Work out the finished part from the listing and answer in its coordinate system (mm). A direction names the side the tool comes from. Coordinates: 2 decimals unless noted, no trailing zeros. Order: outer loops, then holes, each group sorted by start corner. A loop starts at its lowest first (then second) coordinate and runs counter-clockwise, first axis right, second up. Notation, with made-up numbers: M -23.75,82 L 9.25,82 A19 cw 9.25,97 Z; hole C -19,31 d8. An arc over 180 degrees is marked long. Use a Markdown table: item, result. Add a question column.
from build123d import *

# Parameters (mm, degrees)
SKETCH1_W                                  = 200
SKETCH1_H                                  = 400
BOSS_EXTRUDE1_DEPTH                        = 60
SKETCH2_R                                  = 15
CUT_EXTRUDE1_DEPTH                         = 452.220566907
SKETCH3_W                                  = 30
SKETCH3_H                                  = 90
CUT_EXTRUDE2_DEPTH                         = 452.220566907
MIRROR1_AT_THE_SECOND_PLANE_COPY_1_SKETC_W = 30
MIRROR1_AT_THE_SECOND_PLANE_COPY_1_SKETC_H = 90
MIRROR1_AT_THE_SECOND_PLANE_COPY_1_DEPTH   = 452.220566907
FILLET1_R                                  = 10
FILLET2_R                                  = 10


with BuildPart() as part:
    # Sketch1 → Boss-Extrude1 (new body)
    with BuildSketch(Plane.XY):
        with Locations((100, 200)):
            Rectangle(SKETCH1_W, SKETCH1_H)
    extrude(amount=BOSS_EXTRUDE1_DEPTH)

    # Sketch2 → Cut-Extrude1 (cut, through all)
    with BuildSketch(Plane(origin=(200, 0, 0), x_dir=(0, 0, -1), z_dir=(1, 0, 0))):
        with Locations(Location((-30, 40, 0), (0, 0, 90))):
            Circle(SKETCH2_R)
        with Locations(Location((-30, 360, 0), (0, 0, 90))):
            Circle(SKETCH2_R)
    extrude(amount=-CUT_EXTRUDE1_DEPTH, mode=Mode.SUBTRACT)

    # Sketch3 → Cut-Extrude2 (cut, through all)
    with BuildSketch(Plane(origin=(0, 0, 0), x_dir=(-1, 0, 0), z_dir=(0, 0, -1))):
        with Locations((-15, 45)):
            Rectangle(SKETCH3_W, SKETCH3_H)
    cut_extrude2 = extrude(amount=-CUT_EXTRUDE2_DEPTH, mode=Mode.SUBTRACT)

    # Mirror1: Cut-Extrude2 across plane
    add(cut_extrude2.mirror(Plane(origin=(100, 0, 0), x_dir=(0, 0, 1), z_dir=(1, 0, 0))), mode=Mode.SUBTRACT)

    # Mirror1 at the second plane: Cut-Extrude2 across plane
    add(cut_extrude2.mirror(Plane.ZX.offset(200)), mode=Mode.SUBTRACT)

    # Mirror1 at the second plane copy 1 sketc → Mirror1 at the second plane copy 1 (cut, through all)
    with BuildSketch(Plane(origin=(200, 400, 0), x_dir=(1, 0, 0), z_dir=(0, 0, -1))):
        with Locations((-15, 45)):
            Rectangle(MIRROR1_AT_THE_SECOND_PLANE_COPY_1_SKETC_W, MIRROR1_AT_THE_SECOND_PLANE_COPY_1_SKETC_H)
    extrude(amount=-MIRROR1_AT_THE_SECOND_PLANE_COPY_1_DEPTH, mode=Mode.SUBTRACT)

    # Fillet1
    fillet1_edges = [part.edges().sort_by_distance(p)[0] for p in [
        (100, 0, 0),
        (0, 90, 30),
        (30, 45, 60),
        (30, 0, 30),
        (15, 90, 60),
        (15, 90, 0),
        (30, 45, 0),
        (0, 200, 0),
        (0, 200, 60),
        (30, 355, 0),
        (15, 310, 0),
        (0, 310, 30),
        (30, 400, 30),
        (15, 310, 60),
        (30, 355, 60),
        (100, 400, 0),
    ]]
    fillet(fillet1_edges, radius=FILLET1_R)

    # Fillet2
    # the kernel refuses this fillet: 10 mm, written as the material it takes off along each edge
    with BuildSketch(Plane(origin=(40, 10, 50), x_dir=(0, -1, 0), z_dir=(0, 0, 1))) as fillet2_piece_1_section:
        Polygon((0, 0), (FILLET2_R, 0), (FILLET2_R, -FILLET2_R), (0, -FILLET2_R), align=None)
    fillet2_piece_1 = extrude(amount=FILLET2_R, mode=Mode.PRIVATE)
    fillet2_piece_1 = fillet2_piece_1 - Plane(origin=(40, 10, 50), x_dir=(0.7071067811865476, 0.7071067811865475, 0), z_dir=(0, 0, 1)) * Sphere(FILLET2_R, mode=Mode.PRIVATE)
    add(fillet2_piece_1, mode=Mode.SUBTRACT)
    with BuildSketch(Plane(origin=(190, 300, 50), x_dir=(1, 0, 0), z_dir=(0, 0, 1))) as fillet2_piece_2_section:
        Polygon((0, 0), (FILLET2_R, 0), (FILLET2_R, FILLET2_R), (0, FILLET2_R), align=None)
    fillet2_piece_2 = extrude(amount=FILLET2_R, mode=Mode.PRIVATE)
    fillet2_piece_2 = fillet2_piece_2 - Plane(origin=(190, 300, 50), x_dir=(-0.7071067811865471, -0.707106781186548, 0), z_dir=(0, 0, 1)) * Sphere(FILLET2_R, mode=Mode.PRIVATE)
    add(fillet2_piece_2, mode=Mode.SUBTRACT)
    with BuildSketch(Plane(origin=(190, 100, 50), x_dir=(0, -1, 0), z_dir=(0, 0, 1))) as fillet2_piece_3_section:
        Polygon((0, 0), (FILLET2_R, 0), (FILLET2_R, FILLET2_R), (0, FILLET2_R), align=None)
    fillet2_piece_3 = extrude(amount=FILLET2_R, mode=Mode.PRIVATE)
    fillet2_piece_3 = fillet2_piece_3 - Plane(origin=(190, 100, 50), x_dir=(-0.7071067811865472, 0.7071067811865478, 0), z_dir=(0, 0, 1)) * Sphere(FILLET2_R, mode=Mode.PRIVATE)
    add(fillet2_piece_3, mode=Mode.SUBTRACT)
    with BuildSketch(Plane(origin=(160, 10, 50), x_dir=(0, -1, 0), z_dir=(1, 0, 0))) as fillet2_piece_4_section:
        Polygon((0, 0), (FILLET2_R, 0), (FILLET2_R, -FILLET2_R), (0, -FILLET2_R), align=None)
    fillet2_piece_4 = extrude(amount=FILLET2_R, mode=Mode.PRIVATE)
    fillet2_piece_4 = fillet2_piece_4 - Plane(origin=(160, 10, 50), x_dir=(0, 0.7071067811865475, -0.7071067811865475), z_dir=(1, 0, 0)) * Sphere(FILLET2_R, mode=Mode.PRIVATE)
    add(fillet2_piece_4, mode=Mode.SUBTRACT)
    with BuildSketch(Plane(origin=(170, 10, 10), x_dir=(0, 0, -1), z_dir=(0, 1, 0))) as fillet2_piece_5:
        with BuildLine():
            CenterArc((10 - FILLET2_R, FILLET2_R), FILLET2_R, 270, 90)
            Line((10, FILLET2_R), (10, 0))
            Line((10, 0), (10 - FILLET2_R, 0))
        make_face()
    revolve(axis=Axis((170, 10, 10), (-1, 0, 0)), revolution_arc=90, mode=Mode.SUBTRACT)
    with BuildSketch(Plane(origin=(170, 390, 10), x_dir=(0, 0, -1), z_dir=(0, -1, 0))) as fillet2_piece_6:
        with BuildLine():
            CenterArc((10 - FILLET2_R, -FILLET2_R), FILLET2_R, 0, 90)
            Line((10, -FILLET2_R), (10, 0))
            Line((10, 0), (10 - FILLET2_R, 0))
        make_face()
    revolve(axis=Axis((170, 390, 10), (1, 0, 0)), revolution_arc=90, mode=Mode.SUBTRACT)
    with BuildSketch(Plane(origin=(200, 335, 0), x_dir=(-1, 0, 0), z_dir=(0, -1, 0))) as fillet2_piece_7:
        with BuildLine():
            CenterArc((FILLET2_R, -FILLET2_R), FILLET2_R, 90, 90)
            Line((0, -FILLET2_R), (0, 0))
            Line((0, 0), (FILLET2_R, 0))
        make_face()
    extrude(amount=270, mode=Mode.SUBTRACT)
    with BuildSketch(Plane(origin=(200, 300, 60), x_dir=(-1, 0, 0), z_dir=(0, -1, 0))) as fillet2_piece_8:
        with BuildLine():
            CenterArc((FILLET2_R, FILLET2_R), FILLET2_R, 180, 90)
            Line((0, FILLET2_R), (0, 0))
            Line((0, 0), (FILLET2_R, 0))
        make_face()
    extrude(amount=200, mode=Mode.SUBTRACT)
    with BuildSketch(Plane(origin=(170, 90, 0), x_dir=(-1, 0, 0), z_dir=(0, -1, 0))) as fillet2_piece_9:
        with BuildLine():
            CenterArc((FILLET2_R, -FILLET2_R), FILLET2_R, 90, 90)
            Line((0, -FILLET2_R), (0, 0))
            Line((0, 0), (FILLET2_R, 0))
        make_face()
    extrude(amount=80, mode=Mode.SUBTRACT)
    with BuildSketch(Plane(origin=(200, 90, -25), x_dir=(-1, 0, 0), z_dir=(0, 0, 1)), Plane(origin=(200, 310, -25), x_dir=(0, -1, 0), z_dir=(0, 0, 1)), Plane(origin=(170, 400, 10), x_dir=(0, -1, 0), z_dir=(0, 0, 1))) as fillet2_piece_10:
        with BuildLine():
            CenterArc((FILLET2_R, -FILLET2_R), FILLET2_R, 90, 90)
            Line((0, -FILLET2_R), (0, 0))
            Line((0, 0), (FILLET2_R, 0))
        make_face()
    extrude(amount=75, mode=Mode.SUBTRACT)
    with BuildSketch(Plane(origin=(170, 0, 10), x_dir=(0, 1, 0), z_dir=(0, 0, 1))) as fillet2_piece_11:
        with BuildLine():
            CenterArc((FILLET2_R, FILLET2_R), FILLET2_R, 180, 90)
            Line((0, FILLET2_R), (0, 0))
            Line((0, 0), (FILLET2_R, 0))
        make_face()
    extrude(amount=40, mode=Mode.SUBTRACT)
    with BuildSketch(Plane(origin=(190, 90, 60), x_dir=(0, 1, 0), z_dir=(-1, 0, 0))) as fillet2_piece_12:
        with BuildLine():
            CenterArc((FILLET2_R, FILLET2_R), FILLET2_R, 180, 90)
            Line((0, FILLET2_R), (0, 0))
            Line((0, 0), (FILLET2_R, 0))
        make_face()
    extrude(amount=20, mode=Mode.SUBTRACT)
    with BuildSketch(Plane(origin=(170, 90, 60), x_dir=(-1, 0, 0), z_dir=(0, -1, 0)), Plane(origin=(170, 310, 0), x_dir=(-1, 0, 0), z_dir=(0, 1, 0))) as fillet2_piece_13:
        with BuildLine():
            CenterArc((FILLET2_R, FILLET2_R), FILLET2_R, 180, 90)
            Line((0, FILLET2_R), (0, 0))
            Line((0, 0), (FILLET2_R, 0))
        make_face()
    extrude(amount=80, mode=Mode.SUBTRACT)
    with BuildSketch(Plane(origin=(170, 310, 60), x_dir=(-1, 0, 0), z_dir=(0, 1, 0))) as fillet2_piece_14:
        with BuildLine():
            CenterArc((FILLET2_R, -FILLET2_R), FILLET2_R, 90, 90)
            Line((0, -FILLET2_R), (0, 0))
            Line((0, 0), (FILLET2_R, 0))
        make_face()
    extrude(amount=115, mode=Mode.SUBTRACT)
    with BuildSketch(Plane(origin=(190, 310, 60), x_dir=(0, -1, 0), z_dir=(-1, 0, 0))) as fillet2_piece_15:
        with BuildLine():
            CenterArc((FILLET2_R, -FILLET2_R), FILLET2_R, 90, 90)
            Line((0, -FILLET2_R), (0, 0))
            Line((0, 0), (FILLET2_R, 0))
        make_face()
    extrude(amount=20, mode=Mode.SUBTRACT)
    with BuildSketch(Plane(origin=(160, 0, 60), x_dir=(0, 1, 0), z_dir=(-1, 0, 0))) as fillet2_piece_16:
        with BuildLine():
            CenterArc((FILLET2_R, FILLET2_R), FILLET2_R, 180, 90)
            Line((0, FILLET2_R), (0, 0))
            Line((0, 0), (FILLET2_R, 0))
        make_face()
    extrude(amount=120, mode=Mode.SUBTRACT)
    with BuildSketch(Plane(origin=(170, 115, 60), x_dir=(-1, 0, 0), z_dir=(0, -1, 0))) as fillet2_piece_17a_section:
        with BuildLine():
            CenterArc((FILLET2_R, FILLET2_R), FILLET2_R, 180, 90)
            Line((0, FILLET2_R), (0, 0))
            Line((0, 0), (FILLET2_R, 0))
        make_face()
    fillet2_piece_17a = extrude(amount=105, mode=Mode.PRIVATE)
    fillet2_piece_17a = split(fillet2_piece_17a, bisect_by=Plane(origin=(167.736048857, 90, 57.736048857), z_dir=(0, 1, 0)), keep=Keep.TOP, mode=Mode.PRIVATE)
    with BuildSketch(Plane(origin=(190, 90, 60), x_dir=(0, 1, 0), z_dir=(-1, 0, 0))) as fillet2_piece_17b_section:
        with BuildLine():
            CenterArc((FILLET2_R, FILLET2_R), FILLET2_R, 180, 90)
            Line((0, FILLET2_R), (0, 0))
            Line((0, 0), (FILLET2_R, 0))
        make_face()
    fillet2_piece_17b = extrude(amount=45, mode=Mode.PRIVATE)
    fillet2_piece_17b = split(fillet2_piece_17b, bisect_by=Plane(origin=(170, 92.263951143, 57.736048857), z_dir=(-1, 0, 0)), keep=Keep.TOP, mode=Mode.PRIVATE)
    fillet2_piece_17 = fillet2_piece_17a & fillet2_piece_17b
    add(fillet2_piece_17, mode=Mode.SUBTRACT)
    with BuildSketch(Plane(origin=(190, 310, 60), x_dir=(0, -1, 0), z_dir=(-1, 0, 0))) as fillet2_piece_18a_section:
        with BuildLine():
            CenterArc((FILLET2_R, -FILLET2_R), FILLET2_R, 90, 90)
            Line((0, -FILLET2_R), (0, 0))
            Line((0, 0), (FILLET2_R, 0))
        make_face()
    fillet2_piece_18a = extrude(amount=45, mode=Mode.PRIVATE)
    fillet2_piece_18a = split(fillet2_piece_18a, bisect_by=Plane(origin=(170, 307.736048857, 57.736048857), z_dir=(-1, 0, 0)), keep=Keep.TOP, mode=Mode.PRIVATE)
    with BuildSketch(Plane(origin=(170, 285, 60), x_dir=(-1, 0, 0), z_dir=(0, 1, 0))) as fillet2_piece_18b_section:
        with BuildLine():
            CenterArc((FILLET2_R, -FILLET2_R), FILLET2_R, 90, 90)
            Line((0, -FILLET2_R), (0, 0))
            Line((0, 0), (FILLET2_R, 0))
        make_face()
    fillet2_piece_18b = extrude(amount=140, mode=Mode.PRIVATE)
    fillet2_piece_18b = split(fillet2_piece_18b, bisect_by=Plane(origin=(167.736048857, 310, 57.736048857), z_dir=(0, -1, 0)), keep=Keep.TOP, mode=Mode.PRIVATE)
    fillet2_piece_18 = fillet2_piece_18a & fillet2_piece_18b
    add(fillet2_piece_18, mode=Mode.SUBTRACT)


solid = part.part
(1) Given P1, Ø20, axis at y = 61, z = 31.5, coming from the -X side; P2, Ø10, axis at x = 16.5, z = 39, coming from the -Y side; P3, Ø24, axis at x = 176.5, z = 34.5, coming from the +Y side, each flat-ended and moving along its own axis, determine where each tip first touches the part or whether it passes through.
(2) A cutting plane is placed at C-C on z = 30. Write down the section's boundary in (x, y), plus the area to 3 significant figures.
(3) A cutting plane is placed at B-B on x = 155. Write down the section's boundary in (y, z), plus the area to 3 significant figures.
(4) Which of the six approach directions +Z, -Z, +X, -X, +Y, -Y give full straight-line access (tool end or side, diameter ignored) to faces 1 (the cylindrical face through (21.46, 93.01, 2.85)), 2 (the cylindrical face through (21.46, 306.99, 2.85)), 3 (the cylindrical face through (178.54, 92.85, 56.99)), 4 (the flat face through (30, 342, 30)), 5 (the cylindrical face through (167.15, 349.44, 3.01))?
(5) A cutting plane is placed at D-D on x = 178.5. Write down the section's boundary in (y, z).
(6) A cutting plane is placed at A-A on y = 360. Write down the section's boundary in (x, z), plus the area to 3 significant figures.
(7) The mould has two halves that part along Y. Classify faces 6 (the cylindrical face through (197.15, 201.4, 56.99)), 7 (the flat face through (99, 0, 30)), 8 (the cylindrical face through (100.98, 25.015, 30.66)): pulls with the +Y half, pulls with the -Y half, needs draft (parallel to the pull), parting line crosses it, or undercut.
(8) Straight lines are drawn through the part: line 1 (Z direction, x = 100, y = 360); line 2 (Y direction, x = 47.5, z = 22); line 3 (Y direction, x = 93.5, z = 51). For each, find the intervals that lie inside material, in ascending order.
From the geometry:
| question | item | result |
|---|---|---|
| 1 | P1 | stops at x = 30 |
| 1 | P2 | stops at y = 90 |
| 1 | P3 | stops at y = 398.93 |
| 2 | outline | M 0,100 A10 ccw 10,90 L 30,90 L 30,55 L 170,55 L 170,90 L 190,90 A10 ccw 200,100 L 200,300 A10 ccw 190,310 L 170,310 L 170,345 L 30,345 L 30,310 L 10,310 A10 ccw 0,300 Z; M 30,10 A10 ccw 40,0 L 160,0 A10 ccw 170,10 L 170,25 L 30,25 Z; M 30,375 L 170,375 L 170,390 A10 ccw 160,400 L 40,400 A10 ccw 30,390 Z |
| 2 | area | 60,600 mm2 |
| 3 | outline | M 0,10 A10 ccw 10,0 L 390,0 A10 ccw 400,10 L 400,60 L 10,60 A10 ccw 0,50 Z; hole C 40,30 d30; hole C 360,30 d30 |
| 3 | area | 22,500 mm2 |
| 4 | face 1 | -Z, -X, -Y |
| 4 | face 2 | -Z, -X, +Y |
| 4 | face 3 | +Z, +X, -Y |
| 4 | face 4 | +Z, -Z, -X, +Y |
| 4 | face 5 | -Z, +X, +Y |
| 5 | outline | M 90,0 L 310,0 L 310,50 A10 ccw 300,60 L 100,60 A10 ccw 90,50 Z |
| 6 | outline | M 30,10 A10 ccw 40,0 L 160,0 A10 ccw 170,10 L 170,15 L 30,15 Z; M 30,45 L 170,45 L 170,50 A10 ccw 160,60 L 40,60 A10 ccw 30,50 Z |
| 6 | area | 4,110 mm2 |
| 7 | face 6 | needs draft |
| 7 | face 7 | pulls with the -Y half |
| 7 | face 8 | undercut |
| 8 | line 1 | z = 0 to 15, 45 to 60 |
| 8 | line 2 | y = 0 to 27.31, 52.69 to 347.31, 372.69 to 400 |
| 8 | line 3 | y = 0.05 to 400 |
